from build123d import *

# Parameters (mm, degrees)
SKETCH_1_R          = 11
EXTRUDE_1_DEPTH     = 9
SKETCH_2_R          = 0.5
CUT_EXTRUDE_1_DEPTH = 18.972200756
SKETCH_3_R          = 16.549134696
SKETCH_3_R_2        = 9.45
CUT_EXTRUDE_2_DEPTH = 7
SKETCH_4_W          = 2.2
SKETCH_4_H          = 1.7
SKETCH_5_R          = 3
CUT_EXTRUDE_3_DEPTH = 7
SKETCH_7_R          = 1.25
CUT_EXTRUDE_5_DEPTH = 2.5
CUT_EXTRUDE_START   = -1.5
SKETCH_8_R          = 1.25
CUT_EXTRUDE_6_DEPTH = 1.5
SKETCH_9_R          = 4
CUT_EXTRUDE_7_DEPTH = 2
CHAMFER_1_SIZE      = 0.5


with BuildPart() as part:
    # 草图1 → 凸台-拉伸1 (new body)
    with BuildSketch(Plane(origin=(0, 0, 0), x_dir=(1, 0, 0), z_dir=(0, 1, 0))):
        with Locations(Location((0, 0, 0), (0, 0, 270))):
            Circle(SKETCH_1_R)
    extrude(amount=EXTRUDE_1_DEPTH)

    # 草图2 → 切除-拉伸1 (cut, through all)
    with BuildSketch(Plane(origin=(0, 9, 0), x_dir=(1, 0, 0), z_dir=(0, 1, 0))):
        with Locations(Location((-5.5, 0, 0), (0, 0, 270))):
            Circle(SKETCH_2_R)
        with Locations(Location((5.5, 0, 0), (0, 0, 270))):
            Circle(SKETCH_2_R)
    extrude(amount=-CUT_EXTRUDE_1_DEPTH, mode=Mode.SUBTRACT)

    # 草图3 → 切除-拉伸2 (cut)
    with BuildSketch(Plane.XZ):
        Circle(SKETCH_3_R)
        with Locations(Location((0, 0, 0), (0, 0, 270))):
            Circle(SKETCH_3_R_2, mode=Mode.SUBTRACT)
    extrude(amount=-CUT_EXTRUDE_2_DEPTH, mode=Mode.SUBTRACT)

    # 草图4 → 切除-旋转1 (revolve, cut)
    with BuildSketch(Plane.XY, mode=Mode.PRIVATE) as cut_revolve_1_sk:
        with Locations((-9.45, 5.05)):
            Rectangle(SKETCH_4_W, SKETCH_4_H)
        with Locations((-9.45, 2.35)):
            Rectangle(SKETCH_4_W, SKETCH_4_H)
    revolve(cut_revolve_1_sk.sketch.rotate(Axis((0, 0, 0), (0, 1, 0)), 270), axis=Axis((0, 0, 0), (0, 1, 0)), mode=Mode.SUBTRACT)

    # 草图5 → 切除-拉伸3 (cut)
    with BuildSketch(Plane.XZ):
        with Locations(Location((0, 0, 0), (0, 0, 270))):
            Circle(SKETCH_5_R)
    extrude(amount=-CUT_EXTRUDE_3_DEPTH, mode=Mode.SUBTRACT)

    # 草图7 → 切除-拉伸5 (cut)
    with BuildSketch(Plane(origin=(0, 9, 0), x_dir=(1, 0, 0), z_dir=(0, 1, 0))):
        with Locations(Location((-5.5, 0, 0), (0, 0, 270))):
            Circle(SKETCH_7_R)
        with Locations(Location((5.5, 0, 0), (0, 0, 270))):
            Circle(SKETCH_7_R)
    extrude(amount=-CUT_EXTRUDE_5_DEPTH, mode=Mode.SUBTRACT)

    # 草图8 → 切除-拉伸6 (cut)
    with BuildSketch(Plane.XZ.offset(CUT_EXTRUDE_START)):
        with Locations(Location((-5.5, 0, 0), (0, 0, 90))):
            Circle(SKETCH_8_R)
        with Locations(Location((5.5, 0, 0), (0, 0, 90))):
            Circle(SKETCH_8_R)
    extrude(amount=CUT_EXTRUDE_6_DEPTH, mode=Mode.SUBTRACT)

    # 草图9 → 切除-拉伸7 (cut)
    with BuildSketch(Plane.XZ):
        with Locations(Location((0, 0, 0), (0, 0, 270))):
            Circle(SKETCH_9_R)
    extrude(amount=-CUT_EXTRUDE_7_DEPTH, mode=Mode.SUBTRACT)

    # 倒角1
    chamfer_1_edges = [part.edges().sort_by_distance(p)[0] for p in [
        (0, 0, 9.45),
    ]]
    chamfer(chamfer_1_edges, length=CHAMFER_1_SIZE)


solid = part.part
The model under review builds one solid part; all positions refer to its coordinate system, in mm. A direction names the side the tool comes from. Give positions to 0.01 mm unless a question says otherwise; leave off trailing zeros. Loops run counter-clockwise (first coordinate to the right, second up) from the corner with the lowest first, then second, coordinate; pieces in that order, holes last. Notation, with made-up numbers: (36.25, 49) -> (42.25, 49) arc R25 cw to (42.25, 86) -> close; hole circle Ø5 at (79, 47.25). An arc over 180 degrees is marked (long way). Write each question's results on one line, items separated by ' | '.
1) Insertion check: pin 1 Ø2 at (x, z) = (-5.5, 0) entering from +Y; pin 2 Ø1 at (x, y) = (5.5, 7.5) entering from +Z; pin 3 Ø3 at (x, z) = (5, -0.5) entering from +Y; pin 4 Ø0.8 at (x, z) = (5.5, -0.5) entering from -Y. Each pin has a flat end and moves straight along its axis. Give the tip position at first contact, or say it passes through.
Conclusion:
pin 1: stops at y = 6.5 | pin 2: stops at z = 9.8 | pin 3: stops at y = 9 | pin 4: stops at y = 1.5
2) For line 1 along X through (y, z) = (8, 0); line 2 along Y through (x, z) = (7.75, -3.25); line 3 along Y through (x, z) = (1, 2), list the stretches that pass through material, from the lowest coordinate up. Write a range as from..to.
Conclusion:
line 1: x = -11..-6.75, -4.25..4.25, 6.75..11 | line 2: y = 0..1.5, 3.2..4.2, 5.9..9 | line 3: y = 7..9
3) Tool access review of faces 4 (the face through (2.839, 0.993, -9.014)), 5 (the face through (8, 1.5, -3)), 6 (the face through (-6.72, 7.77, -0.27)), 7 (the face through (-10.74, 7.99, -2.38)): name each direction out of +Z, -Z, +X, -X, +Y, -Y from which nothing blocks a thin tool from reaching the whole face with its end or side.
Conclusion:
face 4: -Y | face 5: none | face 6: +Y | face 7: +Y, -Y
4) Draft analysis for pull direction X (two halves, no side actions). For faces 1 (the face through (0.9, 4.46, -2.86)), 2 (the face through (8, 4.2, -3)), 3 (the face through (-2.508, 5.062, -7.964)), state which applies: pulls with the +X half, pulls with the -X half, needs draft (parallel to the pull), parting line crosses it, or undercut.
Conclusion:
face 1: undercut | face 2: needs draft | face 3: parting line crosses it
5) Take a section at A-A, the plane y = 2.75. Give the boundary of the cut face in (x, z), plus the area to 3 significant figures.
Conclusion:
outline: circle Ø16.7 at (0, 0); hole circle Ø1 at (-5.5, 0); hole circle Ø6 at (0, 0); hole circle Ø1 at (5.5, 0) | area: 189 mm^2
6) Take a section at C-C, the plane z = 0. Count the separate pieces of the cut face and the enclosed holes in it, plus the area to 3 significant figures.
Conclusion:
separate pieces: 3 | enclosed holes: 0 | area: 92.6 mm^2
